```python
from build123d import *

# Parameters (mm, degrees)
SKETCH_1_W          = 100
SKETCH_1_H          = 15
EXTRUDE_1_DEPTH     = 3
SKETCH_2_W          = 32
SKETCH_2_H          = 35
EXTRUDE_2_DEPTH     = 3
SKETCH_3_R          = 1.6
CUT_EXTRUDE_1_DEPTH = 54.058929503
SKETCH_4_R          = 2.1
CUT_EXTRUDE_2_DEPTH = 54.058929503
FILLET_1_R          = 4
FILLET_2_R          = 2


with BuildPart() as part:
    # 草图1 → 凸台-拉伸1 (new body)
    with BuildSketch(Plane(origin=(0, 0, 0), x_dir=(1, 0, 0), z_dir=(0, 1, 0))):
        Rectangle(SKETCH_1_W, SKETCH_1_H)
    extrude(amount=EXTRUDE_1_DEPTH)

    # 草图2 → 凸台-拉伸2 (add)
    with BuildSketch(Plane(origin=(0, 3, 0), x_dir=(1, 0, 0), z_dir=(0, 1, 0))):
        Rectangle(SKETCH_2_W, SKETCH_2_H)
    extrude(amount=-EXTRUDE_2_DEPTH)

    # 草图3 → 切除-拉伸1 (cut, through all)
    with BuildSketch(Plane(origin=(0, 3, 0), x_dir=(1, 0, 0), z_dir=(0, 1, 0))):
        with Locations(Location((-42.5, 3.75, 0), (0, 0, 270))):
            Circle(SKETCH_3_R)
        with Locations(Location((-42.5, -3.75, 0), (0, 0, 90))):
            Circle(SKETCH_3_R)
        with Locations(Location((-27.5, -3.75, 0), (0, 0, 270))):
            Circle(SKETCH_3_R)
        with Locations(Location((-27.5, 3.75, 0), (0, 0, 90))):
            Circle(SKETCH_3_R)
        with Locations(Location((42.5, -3.75, 0), (0, 0, 270))):
            Circle(SKETCH_3_R)
        with Locations(Location((42.5, 3.75, 0), (0, 0, 90))):
            Circle(SKETCH_3_R)
        with Locations(Location((27.5, -3.75, 0), (0, 0, 90))):
            Circle(SKETCH_3_R)
        with Locations(Location((27.5, 3.75, 0), (0, 0, 270))):
            Circle(SKETCH_3_R)
    extrude(amount=-CUT_EXTRUDE_1_DEPTH, mode=Mode.SUBTRACT)

    # 草图4 → 切除-拉伸2 (cut, through all)
    with BuildSketch(Plane(origin=(0, 3, 0), x_dir=(1, 0, 0), z_dir=(0, 1, 0))):
        with Locations(Location((-10.5, 12.5, 0), (0, 0, 270))):
            Circle(SKETCH_4_R)
        with Locations(Location((-10.5, -12.5, 0), (0, 0, 90))):
            Circle(SKETCH_4_R)
        with Locations(Location((10.5, -12.5, 0), (0, 0, 270))):
            Circle(SKETCH_4_R)
        with Locations(Location((10.5, 12.5, 0), (0, 0, 90))):
            Circle(SKETCH_4_R)
    extrude(amount=-CUT_EXTRUDE_2_DEPTH, mode=Mode.SUBTRACT)

    # 圆角1
    fillet_1_edges = [part.edges().sort_by_distance(p)[0] for p in [
        (-16, 1.5, 17.5),
        (16, 1.5, -17.5),
        (-16, 1.5, -7.5),
        (-16, 1.5, 7.5),
        (-16, 1.5, -17.5),
        (16, 1.5, -7.5),
        (16, 1.5, 7.5),
        (16, 1.5, 17.5),
    ]]
    fillet(fillet_1_edges, radius=FILLET_1_R)

    # 圆角2
    fillet_2_edges = [part.edges().sort_by_distance(p)[0] for p in [
        (50, 1.5, 7.5),
        (-50, 1.5, 7.5),
        (-50, 1.5, -7.5),
        (50, 1.5, -7.5),
    ]]
    fillet(fillet_2_edges, radius=FILLET_2_R)


solid = part.part
```
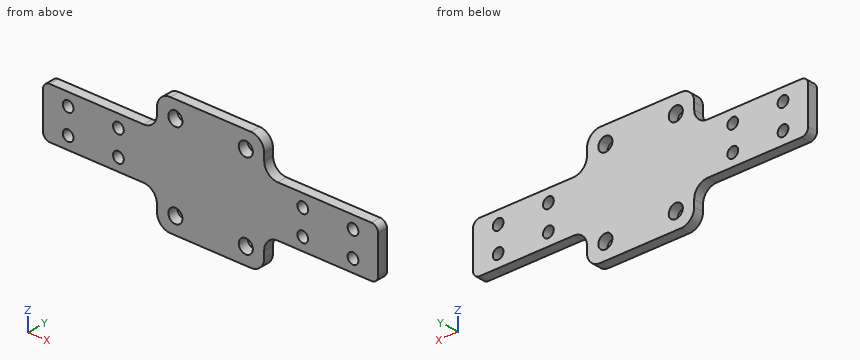
The model under review builds one solid part; all positions refer to its coordinate system, in mm. Round coordinates to 2 decimals unless told otherwise and drop trailing zeros. Loops run counter-clockwise (first coordinate to the right, second up) from the corner with the lowest first, then second, coordinate; pieces in that order, holes last. Notation, with made-up numbers: (46, 15) -> (90, 15) arc R17 ccw to (90, 20) -> close; hole circle Ø2 at (-38.5, 49). An arc over 180 degrees is marked (long way). Answer as a JSON object with one key per item and string values. Group by question number.
1) We need section B-B on x = -27.5. Write out the cut boundary in (y, z), then the cut area to 3 significant figures.
2) For pin 1 Ø0.6 at (y, z) = (2, 12) entering from -X; pin 2 Ø3 at (x, z) = (-14.5, 9.5) entering from -Y; pin 3 Ø1.5 at (x, y) = (-27, 1) entering from -Z; pin 4 Ø0.6 at (y, z) = (1.5, 12) entering from +X, all flat-tipped, find the tip position at first contact; note any pin that passes through.
3) We need section A-A on z = -12.5. Write out the cut boundary in (x, y).
4) We need section D-D on y = 1.7. Give the number of separate pieces and of enclosed holes in the cut face, then the cut area to 3 significant figures.
5) We need section C-C on z = -3.75. Write out the cut boundary in (x, y), then the cut area to 3 significant figures.
6) For line 1 (X direction, y = 1.2, z = -3.75); line 2 (Z direction, x = -43.5, y = 1.45); line 3 (Z direction, x = 31, y = 2.35), list the stretches that pass through material, from the lowest coordinate up. Write a range as [from, to].
Result set:
{
 "1": {"outline": "(0, -7.5) -> (3, -7.5) -> (3, -5.35) -> (0, -5.35) -> close; (0, -2.15) -> (3, -2.15) -> (3, 2.15) -> (0, 2.15) -> close; (0, 5.35) -> (3, 5.35) -> (3, 7.5) -> (0, 7.5) -> close", "area": "25.8 mm²"},
 "2": {"pin 1": "x = -16", "pin 2": "y = 0", "pin 3": "z = -7.5", "pin 4": "x = 16"},
 "3": {"outline": "(-16, 0) -> (-12.6, 0) -> (-12.6, 3) -> (-16, 3) -> close; (-8.4, 0) -> (8.4, 0) -> (8.4, 3) -> (-8.4, 3) -> close; (12.6, 0) -> (16, 0) -> (16, 3) -> (12.6, 3) -> close"},
 "4": {"separate pieces": "1", "enclosed holes": "12", "area": "2,020 mm²"},
 "5": {"outline": "(-50, 0) -> (-44.1, 0) -> (-44.1, 3) -> (-50, 3) -> close; (-40.9, 0) -> (-29.1, 0) -> (-29.1, 3) -> (-40.9, 3) -> close; (-25.9, 0) -> (25.9, 0) -> (25.9, 3) -> (-25.9, 3) -> close; (29.1, 0) -> (40.9, 0) -> (40.9, 3) -> (29.1, 3) -> close; (44.1, 0) -> (50, 0) -> (50, 3) -> (44.1, 3) -> close", "area": "262 mm²"},
 "6": {"line 1": "[-50, -44.1], [-40.9, -29.1], [-25.9, 25.9], [29.1, 40.9], [44.1, 50]", "line 2": "[-7.5, -5], [-2.5, 2.5], [5, 7.5]", "line 3": "[-7.5, 7.5]"}
}
